```python
from build123d import *

# Parameters (mm, degrees)
F0_W     = 145.373996
F0_H     = 82.43306
F1_DEPTH = 55.88
F2_SIZE  = 5.08
F3_T     = -2.54
F5_D     = 38.1


with BuildPart() as f1:
    # F0 (on Top) → F1 (new body)
    with BuildSketch(Plane.XY):
        with Locations((-31.786533, -41.21653)):
            Rectangle(F0_W, F0_H)
    extrude(amount=F1_DEPTH)

    # F2
    f2_edges = [f1.edges().sort_by_distance(p)[0] for p in [
        (-31.786533, -82.43306, 55.88),
        (40.900465, -41.21653, 55.88),
        (-31.786533, 0, 55.88),
        (-104.473531, -41.21653, 55.88),
        (-104.473531, -82.43306, 27.94),
        (40.900465, -82.43306, 27.94),
        (-31.786533, -82.43306, 0),
        (40.900465, 0, 27.94),
        (40.900465, -41.21653, 0),
        (-104.473531, 0, 27.94),
        (-104.473531, -41.21653, 0),
        (-31.786533, 0, 0),
    ]]
    chamfer(f2_edges, length=F2_SIZE)

    # F3
    f3_openings = [f1.faces().sort_by_distance(p)[0] for p in [
        (-31.786533, -41.21653, 0),
    ]]
    offset(amount=F3_T, openings=f3_openings)

    # F5 (through all)
    with Locations(Plane(origin=(0, 0, 53.34), x_dir=(1, 0, 0), z_dir=(0, 0, -1))):
        with Locations((-26.097942, 51.094607)):
            Hole(F5_D / 2)


solid = f1.part
```
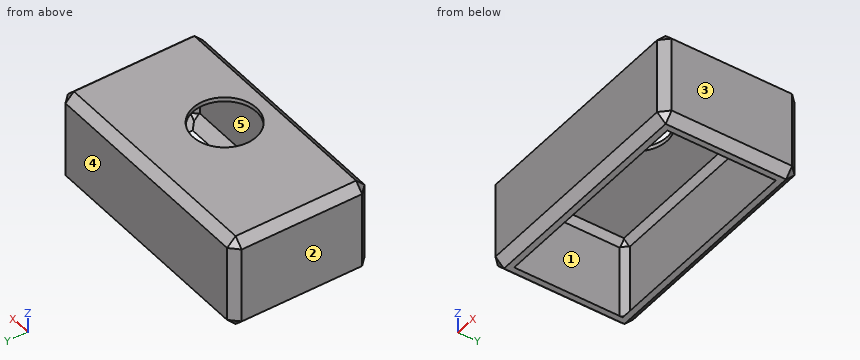
Could you check a few things on this model? Use its own coordinates, in mm. Face numbers are marked on the shaded views. A direction names the side the tool comes from. Coordinates: 2 decimals unless noted, no trailing zeros. Loops run counter-clockwise (first coordinate to the right, second up) from the corner with the lowest first, then second, coordinate; pieces in that order, holes last. Notation, with made-up numbers: M -13,-12 L -8,-12 A21 ccw -8,15 Z; hole C 87.5,44.25 d10. An arc over 180 degrees is marked long. Put each result on its own line as item: value. Start each with the question number.
(1) Thinking about a two-plate mould opening in Y: for the marked faces 3, 4 and 5, which applies, pulls with the +Y half, pulls with the -Y half, needs draft (parallel to the pull), parting line crosses it, or undercut?
(2) Suppose I cut it at A-A on z = 47.5. Please give me the cut outline in (x, y), then the cut area to 3 significant figures.
(3) Will this pin go through, and if not, where does the flat tip stop? P1, Ø1.5, axis at x = -10, y = -16.5, coming from the -Z side.
(4) Suppose I cut it at C-C on x = -33. Please give me the cut outline in (y, z).
(5) Suppose I cut it at B-B on y = -36.5. Please give me the cut outline in (x, z), then the cut area to 3 significant figures.
(6) Suppose I cut it at D-D on x = -67. Please give me the cut outline in (y, z).
(7) For the marked faces 1 and 2, which set-ups out of +Z, -Z, +X, -X, +Y, -Y let a thin tool reach every point of the face, with its end or its side?
(8) I need wall thicknesses on line 1 (Y direction, x = -27, z = 39); line 2 (X direction, y = -11, z = 39.5); line 3 (Z direction, x = -22.5, y = -17). Which ranges of each line are inside material? Lowest first, please. Write a range as from..to.
Solutions:
1. face 3: needs draft
1. face 4: pulls with the +Y half
1. face 5: undercut
2. outline: M -104.47,-77.35 L -99.39,-82.43 L 35.82,-82.43 L 40.9,-77.35 L 40.9,-5.08 L 35.82,0 L -99.39,0 L -104.47,-5.08 Z; hole M -101.93,-76.3 L -98.34,-79.89 L 34.77,-79.89 L 38.36,-76.3 L 38.36,-6.13 L 34.77,-2.54 L -98.34,-2.54 L -101.93,-6.13 Z
2. area: 1,110 mm2
3. P1: stops at z = 53.34
4. outline: M -82.43,5.08 L -77.35,0 L -73.76,0 L -79.89,6.13 L -79.89,49.75 L -76.3,53.34 L -68.85,53.34 L -68.85,55.88 L -77.35,55.88 L -82.43,50.8 Z; M -33.34,53.34 L -6.13,53.34 L -2.54,49.75 L -2.54,6.13 L -8.67,0 L -5.08,0 L 0,5.08 L 0,50.8 L -5.08,55.88 L -33.34,55.88 Z
5. outline: M -104.47,5.08 L -99.39,0 L -95.8,0 L -101.93,6.13 L -101.93,49.75 L -98.34,53.34 L -38.34,53.34 L -38.34,55.88 L -99.39,55.88 L -104.47,50.8 Z; M -13.85,53.34 L 34.77,53.34 L 38.36,49.75 L 38.36,6.13 L 32.23,0 L 35.82,0 L 40.9,5.08 L 40.9,50.8 L 35.82,55.88 L -13.85,55.88 Z
5. area: 577 mm2
6. outline: M -82.43,5.08 L -77.35,0 L -73.76,0 L -79.89,6.13 L -79.89,49.75 L -76.3,53.34 L -6.13,53.34 L -2.54,49.75 L -2.54,6.13 L -8.67,0 L -5.08,0 L 0,5.08 L 0,50.8 L -5.08,55.88 L -77.35,55.88 L -82.43,50.8 Z
7. face 1: none
7. face 2: +Z, -Z, -X, +Y, -Y
8. line 1: y = -82.43..-79.89, -2.54..0
8. line 2: x = -104.47..-101.93, 38.36..40.9
8. line 3: z = 53.34..55.88
